For this review, take the finished solid that the model builds, in its own axes (mm). Give positions to 0.01 mm unless a question says otherwise; leave off trailing zeros. Loops run counter-clockwise (first coordinate to the right, second up) from the corner with the lowest first, then second, coordinate; pieces in that order, holes last. Notation, with made-up numbers: (85, 25) -> (134, 25) arc R31 ccw to (134, 52) -> close; hole circle Ø9 at (1, 30.25). An arc over 180 degrees is marked (long way). Answer as CSV lines item,"result". Start each with the question number.
Item 1: Add section C-C on x = -204. State the section outline as (y, z) points, plus the area to 3 significant figures.
Item 2: Clearance check with a flat-ended pin moving along its axis: P1, Ø5, axis at x = -175, z = 4, coming from the -Y side. State where the tip first meets the part, or that it passes through.
Item 3: Add section D-D on x = 169. State the section outline as (y, z) points.
Item 4: For L1, parallel to Y at x = -180, z = 0.75; L2, parallel to Z at x = -218.5, y = 2.75, list the stretches that pass through material, from the lowest coordinate up. Write a range as from..to.
```python
from build123d import *


with BuildPart() as part:
    # Esquisse1 → Révolution1 (revolve)
    with BuildSketch(Plane.XY, mode=Mode.PRIVATE) as r_volution1_sk:
        Polygon((-250, 0), (-250, 3.2), (-249.2, 4), (-235, 4), (-235, 4.1), (-234.1, 5), (-196, 5), (-196, 5.1), (-195.1, 6), (199, 6), (200, 5), (200, 4), (207, 4), (207, 3.8), (207.9, 3.8), (207.9, 4), (209.2, 4), (210, 3.2), (210, 0), align=None)
    revolve(r_volution1_sk.sketch.rotate(Axis((-511.970894611, 0, 0), (1, 0, 0)), 180), axis=Axis((-511.970894611, 0, 0), (1, 0, 0)))


solid = part.part
```
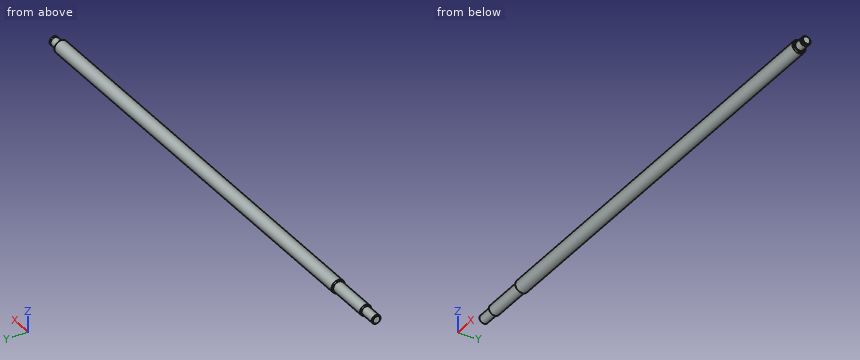
Computed values:
1,outline,"circle Ø10 at (0, 0)"
1,area,"78.5 mm²"
2,P1,"y = -5.81"
3,outline,"circle Ø12 at (0, 0)"
4,L1,"-5.95..5.95"
4,L2,"-4.18..4.18"
